The listing builds one solid part. Answer for the finished solid, in the listing's coordinates (mm). A direction names the side the tool comes from. Give positions to 0.01 mm unless a question says otherwise; leave off trailing zeros. Loops run counter-clockwise (first coordinate to the right, second up) from the corner with the lowest first, then second, coordinate; pieces in that order, holes last. Notation, with made-up numbers: (83.25, 10.25) -> (132.25, 10.25) arc R25 cw to (132.25, 47.25) -> close; hole circle Ø4 at (-20, 28.25). An arc over 180 degrees is marked (long way). One line per question, with ' | ' between items. Start each with the question number.
from build123d import *

# Parameters (mm, degrees)
SKETCH1_R           = 2
SKETCH1_R_2         = 3.125
BOSS_EXTRUDE1_DEPTH = 9.525
FILLET1_R           = 5


with BuildPart() as part:
    # Sketch1 → Boss-Extrude1 (new body)
    with BuildSketch(Plane(origin=(0, 0, 0), x_dir=(1, 0, 0), z_dir=(0, 1, 0))):
        Polygon((-12.7, 5.628932188), (-48.106601718, 41.035533906), (-41.035533906, 48.106601718), (-5.628932188, 12.7), (-5.628932188, 31.75), (5.628932188, 31.75), (5.628932188, 12.7), (41.035533906, 48.106601718), (48.106601718, 41.035533906), (12.7, 5.628932188), (12.7, -5.628932188), (48.106601718, -41.035533906), (41.035533906, -48.106601718), (5.628932188, -12.7), (5.628932188, -31.75), (-5.628932188, -31.75), (-5.628932188, -12.7), (-41.035533906, -48.106601718), (-48.106601718, -41.035533906), (-12.7, -5.628932188), align=None)
        with Locations(Location((37.5, 37.5, 0), (0, 0, 90))):
            Circle(SKETCH1_R, mode=Mode.SUBTRACT)
        with Locations(Location((37.5, -37.5, 0), (0, 0, 90))):
            Circle(SKETCH1_R, mode=Mode.SUBTRACT)
        with Locations(Location((-37.5, -37.5, 0), (0, 0, 90))):
            Circle(SKETCH1_R, mode=Mode.SUBTRACT)
        with Locations(Location((-37.5, 37.5, 0), (0, 0, 90))):
            Circle(SKETCH1_R, mode=Mode.SUBTRACT)
        with Locations(Location((0, 0, 0), (0, 0, 90))):
            Circle(SKETCH1_R_2, mode=Mode.SUBTRACT)
        with Locations(Location((0, 25.4, 0), (0, 0, 90))):
            Circle(SKETCH1_R_2, mode=Mode.SUBTRACT)
        with Locations(Location((0, -25.4, 0), (0, 0, 90))):
            Circle(SKETCH1_R_2, mode=Mode.SUBTRACT)
    extrude(amount=BOSS_EXTRUDE1_DEPTH)

    # Fillet1
    fillet1_edges = [part.edges().sort_by_distance(p)[0] for p in [
        (12.7, 4.7625, -5.628932188),
        (12.7, 4.7625, 5.628932188),
        (48.106601718, 4.7625, 41.035533906),
        (41.035533906, 4.7625, 48.106601718),
        (-41.035533906, 4.7625, 48.106601718),
        (-48.106601718, 4.7625, 41.035533906),
        (-12.7, 4.7625, 5.628932188),
        (-48.106601718, 4.7625, -41.035533906),
        (-41.035533906, 4.7625, -48.106601718),
        (41.035533906, 4.7625, -48.106601718),
        (48.106601718, 4.7625, -41.035533906),
        (-12.7, 4.7625, -5.628932188),
        (-5.628932188, 4.7625, 31.75),
        (-5.628932188, 4.7625, 12.7),
        (5.628932188, 4.7625, 12.7),
        (5.628932188, 4.7625, -12.7),
        (5.628932188, 4.7625, -31.75),
        (-5.628932188, 4.7625, -31.75),
        (-5.628932188, 4.7625, -12.7),
        (5.628932188, 4.7625, 31.75),
    ]]
    fillet(fillet1_edges, radius=FILLET1_R - 0.0001)  # a hair under: the kernel refuses the full size


solid = part.part
1. Each of these flat-tipped pins is pushed along its axis until it touches: pin 1 Ø5.5 at (y, z) = (4.5, -0.5) entering from -X; pin 2 Ø4 at (x, y) = (35, 3.5) entering from +Z; pin 3 Ø1.5 at (x, y) = (-23, 6.5) entering from -Z; pin 4 Ø10 at (x, z) = (0, 0) entering from -Y. Where does it stop, or does it pass through?
2. Straight lines are drawn through the part: L1, parallel to X at y = 7.5, z = 36; L2, parallel to Z at x = -37.5, y = 2; L3, parallel to X at y = 2, z = -25.4 (3 decimals). For each, find the intervals that lie inside material, in ascending order.
3. For faces 1 (the flat face through (29.58, 4.7, -22.51)), 2 (the flat face through (-26, 4.7, -33.07)), 3 (the flat face through (-12.7, 5, 0)), 4 (the flat face through (-25.67, 4.7, 32.74)), 5 (the cylindrical face through (-0.14, 4.7, 28.52)), determine the directions among +Z, -Z, +X, -X, +Y, -Y from which every point of the face is accessible in a straight line to the end or side of a thin tool.
4. The part is cut by section B-B (z = 0). Write down the section's boundary in (x, y) (3 decimals).
5. The part is cut by section C-C (y = 2.75). Count the separate pieces of the cut face and the enclosed holes in it, plus the area to 3 significant figures.
6. The part is cut by section D-D (x = -7). Write down the section's boundary in (y, z) (3 decimals), plus the area to 3 significant figures.
7. Determine the mould class of faces 6 (the flat face through (29.15, 4.7, 22.08)), 7 (the cylindrical face through (-13.07, 4.83, 5.45)), 8 (the flat face through (5.629, 5, -26)) for opening direction X: released by +X, released by -X, zero draft, split by the parting line, or undercut.
8. The part is cut by section A-A (x = 32). Write down the section's boundary in (y, z) (3 decimals).
Check sheet entries:
1) pin 1: stops at x = -12.7 | pin 2: stops at z = 44.07 | pin 3: stops at z = -30.82 | pin 4: stops at y = 0
2) L1: x = -43.07 to -38.82, -36.18 to -28.93, 28.93 to 36.18, 38.82 to 43.07 | L2: z = -44.57 to -39.5, -35.5 to -30.43, 30.43 to 35.5, 39.5 to 44.57 | L3: x = -32.471 to -18.329, -5.629 to -3.125, 3.125 to 5.629, 18.329 to 32.471
3) face 1: +X, +Y, -Y | face 2: -Z, +Y, -Y | face 3: -X, +Y, -Y | face 4: +Z, +Y, -Y | face 5: +Y, -Y
4) outline: (-12.7, 0) -> (-3.125, 0) -> (-3.125, 9.525) -> (-12.7, 9.525) -> close; (3.125, 0) -> (12.7, 0) -> (12.7, 9.525) -> (3.125, 9.525) -> close
5) separate pieces: 1 | enclosed holes: 7 | area: 2,900 mm^2
6) outline: (0, -21.331) -> (9.525, -21.331) -> (9.525, 21.331) -> (0, 21.331) -> close | area: 406 mm^2
7) face 6: released by +X | face 7: released by -X | face 8: undercut
8) outline: (0, -39.071) -> (9.525, -39.071) -> (9.525, -24.929) -> (0, -24.929) -> close; (0, 24.929) -> (9.525, 24.929) -> (9.525, 39.071) -> (0, 39.071) -> close
